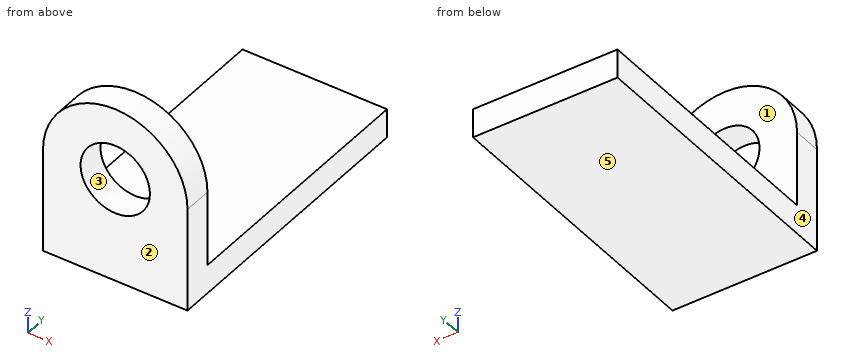
```python
from build123d import *

# Parameters (mm, degrees)
SKETCH_W     = 25
SKETCH_H     = 50
PAD_DEPTH    = 5
SKETCH001_R  = 6
PAD001_DEPTH = 5


with BuildPart() as part:
    # Sketch → Pad (new body)
    with BuildSketch(Plane.XY):
        with Locations((12.5, 25)):
            Rectangle(SKETCH_W, SKETCH_H)
    extrude(amount=PAD_DEPTH)

    # Sketch001 (on Face1 of Pad) → Pad001 (join)
    with BuildSketch(Plane.XZ):
        with BuildLine():
            Line((0, 0), (0, 18))
            ThreePointArc((25, 18), (12.5, 30.5), (0, 18))
            Line((25, 0), (25, 18))
            Line((0, 0), (25, 0))
        make_face()
        with Locations((12.5, 18)):
            Circle(SKETCH001_R, mode=Mode.SUBTRACT)
    extrude(amount=-PAD001_DEPTH)


solid = part.part
```
Model file for the job. Use its own axes, mm. Face numbers are marked on the shaded views. A direction names the side the tool comes from. Coordinates: 2 decimals unless noted, no trailing zeros. Loops run counter-clockwise (first coordinate to the right, second up) from the corner with the lowest first, then second, coordinate; pieces in that order, holes last. Notation, with made-up numbers: (40.5, -6) - (82.5, -6) arc R19 cw to (82.5, 19) - close; hole circle Ø10 at (75.5, 0). An arc over 180 degrees is marked (long way). Answer as a JSON object with one key per item and string values. Group by question number.
(1) Flat gauge pins, fed straight in: pin 1 (2 mm diameter, centred on x = 17, y = 41.5, fed in from +Z); pin 2 (10 mm diameter, centred on x = 22, z = 6.5, fed in from -Y); pin 3 (10 mm diameter, centred on x = 7, z = 14.5, fed in from +Y); pin 4 (2 mm diameter, centred on y = 42.5, z = 7, fed in from -X). Where does each tip first touch, or does it go through?
(2) Cut at B-B (z = 13). Give the cut face in (x, y), then the cut area to 3 significant figures.
(3) Cut at A-A (x = 12.5). Give the cut face in (y, z), then the cut area to 4 significant figures.
(4) Cut at C-C (y = 35.5). Give the cut face in (x, z).
(5) Tool access for the marked faces 1 and 2: list every direction of +Z, -Z, +X, -X, +Y, -Y with a clear straight run to the whole face (end or side of a thin tool).
(6) Probe line 1 along Z through (x, y) = (12.5, 3.75); line 2 along Y through (x, z) = (8, 25.5). List the from-to ranges inside material, lowest first.
(7) Two-plate mould, pull along X, no slides. Class the marked faces 3, 4 and 5: released by +X, released by -X, zero draft, split by the parting line, or undercut.
(8) Cut at D-D (x = 1.5). Give the cut face in (y, z).
Geometry says:
{
 "1": {"pin 1": "stops at z = 5", "pin 2": "stops at y = 0", "pin 3": "stops at y = 5", "pin 4": "passes through"},
 "2": {"outline": "(0, 0) - (9.18, 0) - (9.18, 5) - (0, 5) - close; (15.82, 0) - (25, 0) - (25, 5) - (15.82, 5) - close", "area": "91.8 mm^2"},
 "3": {"outline": "(0, 0) - (50, 0) - (50, 5) - (5, 5) - (5, 12) - (0, 12) - close; (0, 24) - (5, 24) - (5, 30.5) - (0, 30.5) - close", "area": "317.5 mm^2"},
 "4": {"outline": "(0, 0) - (25, 0) - (25, 5) - (0, 5) - close"},
 "5": {"face 1": "+Z, +X, -X, +Y", "face 2": "+Z, -Z, +X, -X, -Y"},
 "6": {"line 1": "z = 0 to 12, 24 to 30.5", "line 2": "y = 0 to 5"},
 "7": {"face 3": "undercut", "face 4": "released by -X", "face 5": "zero draft"},
 "8": {"outline": "(0, 0) - (50, 0) - (50, 5) - (5, 5) - (5, 23.94) - (0, 23.94) - close"}
}
